Could you check a few things on this model? Use its own coordinates, in mm. A direction names the side the tool comes from. Give positions to 0.01 mm unless a question says otherwise; leave off trailing zeros. Order: outer loops, then holes, each group sorted by start corner. A loop starts at its lowest first (then second) coordinate and runs counter-clockwise, first axis right, second up.
(1) Imagine slicing it at B-B, the plane x = -17.5. Write out the boundary of the cut face in (y, z), then the cut area to 3 significant figures.
(2) Imagine slicing it at C-C, the plane z = 4.5. Write out the boundary of the cut face in (x, y).
(3) If I drill on probe 1 along Y at (x, z) = (-32, -11); probe 2 along Z at (x, y) = (-11, -22); probe 3 along Z at (x, y) = (-8.5, -17.5), over which ranges is the centre line in solid material (lowest first)?
(4) If we mould it in two halves opening along Z, with no side actions, what happens to faces 4 (the flat face through (-18, -25.4, 8)), 5 (the flat face through (-12, -13, -23.774)), 6 (the flat face through (-18.1, -0.36, 2.93)), 7 (the flat face through (-6.087, -0.356, 3.201))? For each: released by +Z, released by -Z, zero draft, split by the parting line, or undercut.
(5) Will these pins go through, and if not, where does the flat tip stop? pin 1 (2 mm diameter, centred on x = -10, y = 17.5, fed in from -Z); pin 2 (1 mm diameter, centred on y = 1, z = 12, fed in from -X); pin 3 (6 mm diameter, centred on y = 13.5, z = 20.5, fed in from -X).
(6) Imagine slicing it at D-D, the plane z = -14.5. Write out the boundary of the cut face in (x, y), then the cut area to 3 significant figures.
(7) On a 3-axis mill with a long thin cutter (end or side, diameter ignored), from which of +Z, -Z, +X, -X, +Y, -Y can I reach the whole of each face in a straight line? I mean faces 1 (the flat face through (-12, 0, -6.446)), 2 (the cylindrical face through (6.164, 12.522, 7.348)), 3 (the flat face through (-12, -13, 27.026)). Say none if no direction works.
(8) Imagine slicing it at A-A, the plane y = -13.5. Write out the boundary of the cut face in (x, z).
from build123d import *

# Parameters (mm, degrees)
F0_W     = 50.8
F0_H     = 50.8
F0_R     = 19.05
F1_DEPTH = 25.4
F2_DEPTH = 25.4


with BuildPart() as f1:
    # F0 (on Front) → F1 (new body)
    with BuildSketch(Plane.XZ):
        with Locations((-12.006546, 1.62563)):
            Rectangle(F0_W, F0_H)
        with Locations((-12.006546, 1.62563)):
            Circle(F0_R, mode=Mode.SUBTRACT)
        with Locations((-12.006546, 1.62563)):
            Circle(F0_R)
        Polygon((0, -6.445928), (-24.020746, -6.445928), (-12.006546, 12.581361), align=None, mode=Mode.SUBTRACT)
    extrude(amount=F1_DEPTH)

    # F0 (on Front) → F2 (join)
    with BuildSketch(Plane.XZ):
        with Locations((-12.006546, 1.62563)):
            Circle(F0_R)
        Polygon((0, -6.445928), (-24.020746, -6.445928), (-12.006546, 12.581361), align=None, mode=Mode.SUBTRACT)
    extrude(amount=-F2_DEPTH)


solid = f1.part
Answer block:
1. outline: (-25.4, -23.77) - (0, -23.77) - (0, -16.62) - (25.4, -16.62) - (25.4, -6.45) - (-25.4, -6.45) - close; (-25.4, 3.88) - (25.4, 3.88) - (25.4, 19.87) - (0, 19.87) - (0, 27.03) - (-25.4, 27.03) - close
1. area: 1,690 mm2
2. outline: (-37.41, -25.4) - (-17.11, -25.4) - (-17.11, 25.4) - (-30.84, 25.4) - (-30.84, 0) - (-37.41, 0) - close; (-6.91, -25.4) - (13.39, -25.4) - (13.39, 0) - (6.83, 0) - (6.83, 25.4) - (-6.91, 25.4) - close
3. probe 1: y = -25.4 to 0
3. probe 2: z = -23.77 to -6.45, 10.99 to 27.03
3. probe 3: z = -23.77 to -6.45, 7.02 to 27.03
4. face 4: zero draft
4. face 5: released by -Z
4. face 6: undercut
4. face 7: undercut
5. pin 1: stops at z = -17.4
5. pin 2: stops at x = -28.3
5. pin 3: stops at x = -22.54
6. outline: (-37.41, -25.4) - (13.39, -25.4) - (13.39, 0) - (-1.86, 0) - (-1.86, 25.4) - (-22.15, 25.4) - (-22.15, 0) - (-37.41, 0) - close
6. area: 1,810 mm2
7. face 1: +Y, -Y
7. face 2: +Y
7. face 3: +Z, +X, -X, +Y, -Y
8. outline: (-37.41, -23.77) - (13.39, -23.77) - (13.39, 27.03) - (-37.41, 27.03) - close; hole (-24.02, -6.45) - (0, -6.45) - (-12.01, 12.58) - close
